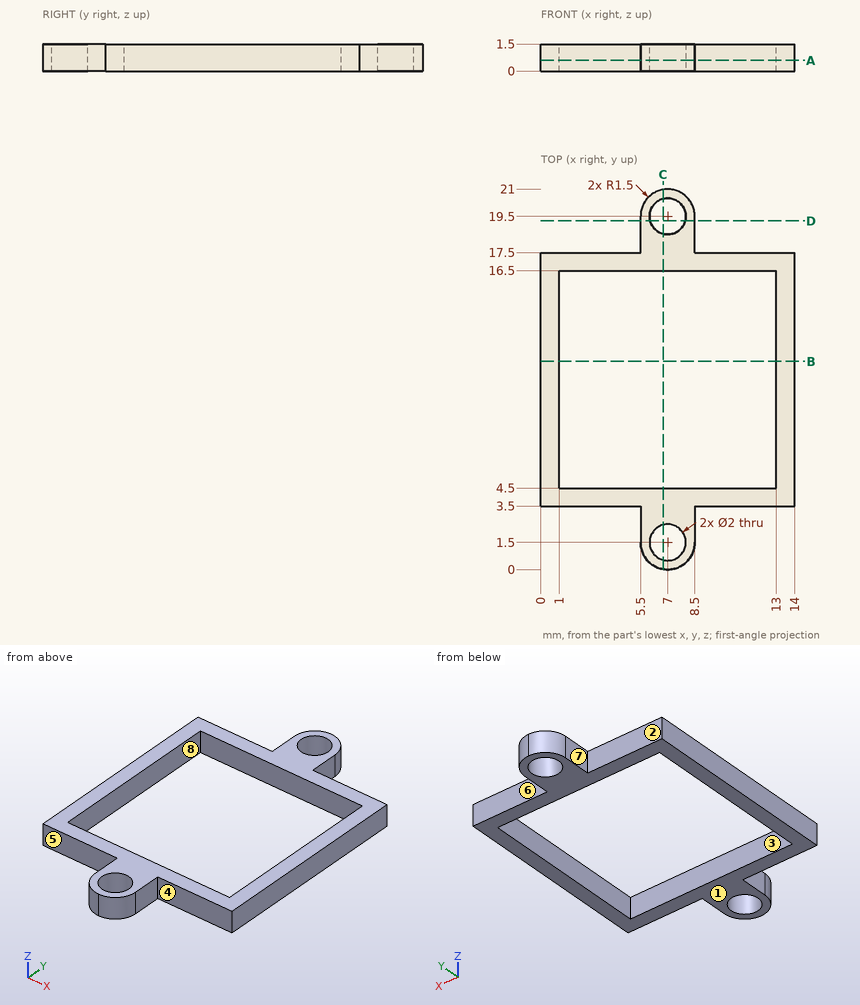
Answer from the drawing. Dimensions are ordinates in mm from the lowest x, y and z of the part. A direction names the side the tool comes from. Round coordinates to 2 decimals unless told otherwise and drop trailing zeros. Loops run counter-clockwise (first coordinate to the right, second up) from the corner with the lowest first, then second, coordinate; pieces in that order, holes last.
(1) Find the intervals of material crossed by L1, parallel to Y at x = 7, z = 0.6; L2, parallel to Y at x = 9.5, z = 0.8; L3, parallel to X at y = 16, z = 0.85, in increasing order.
Computed values:
L1: y = 0 to 0.5, 2.5 to 4.5, 16.5 to 18.5, 20.5 to 21
L2: y = 3.5 to 4.5, 16.5 to 17.5
L3: x = 0 to 1, 13 to 14
(2) The part is cut by section D-D, the plane y = 19.25. Give the vertices of the cut face in (x, z).
Computed values:
outline: (5.5, 0) - (6.03, 0) - (6.03, 1.5) - (5.5, 1.5) - close; (7.97, 0) - (8.5, 0) - (8.5, 1.5) - (7.97, 1.5) - close
(3) The part is cut by section A-A, the plane z = 0.6. Give the vertices of the cut face in (x, y).
Computed values:
outline: (0, 3.5) - (5.5, 3.5) - (5.5, 1.5) arc R1.5 ccw to (8.5, 1.5) - (8.5, 3.5) - (14, 3.5) - (14, 17.5) - (8.5, 17.5) - (8.5, 19.5) arc R1.5 ccw to (5.5, 19.5) - (5.5, 17.5) - (0, 17.5) - close; hole (1, 4.5) - (13, 4.5) - (13, 16.5) - (1, 16.5) - close; hole circle Ø2 at (7, 1.5); hole circle Ø2 at (7, 19.5)
(4) The part is cut by section C-C, the plane x = 6.75. Give the vertices of the cut face in (y, z).
Computed values:
outline: (0.02, 0) - (0.53, 0) - (0.53, 1.5) - (0.02, 1.5) - close; (2.47, 0) - (4.5, 0) - (4.5, 1.5) - (2.47, 1.5) - close; (16.5, 0) - (18.53, 0) - (18.53, 1.5) - (16.5, 1.5) - close; (20.47, 0) - (20.98, 0) - (20.98, 1.5) - (20.47, 1.5) - close
(5) For the marked faces 5, 6, 7 and 8, determine the directions among +Z, -Z, +X, -X, +Y, -Y from which every point of the face is accessible in a straight line to the end or side of a thin tool.
Computed values:
face 5: +Z, -Z, -X, -Y
face 6: +Z, -Z, +X, +Y
face 7: +Z, -Z, -X, +Y
face 8: +Z, -Z
(6) The mould has two halves that part along Y. Classify the marked faces 1, 2, 3 and 4: pulls with the +Y half, pulls with the -Y half, needs draft (parallel to the pull), parting line crosses it, or undercut.
Computed values:
face 1: needs draft
face 2: pulls with the +Y half
face 3: undercut
face 4: pulls with the -Y half
(7) Each of these flat-tipped pins is pushed along its axis until it touches: P1, Ø0.8, axis at x = 4, z = 0.5, coming from the +Y side; P2, Ø0.8, axis at x = 9.5, z = 0.5, coming from the -Y side. Where does it stop, or does it pass through?
Computed values:
P1: stops at y = 17.5
P2: stops at y = 3.5
(8) The part is cut by section B-B, the plane y = 11.5. Give the vertices of the cut face in (x, z).
Computed values:
outline: (0, 0) - (1, 0) - (1, 1.5) - (0, 1.5) - close; (13, 0) - (14, 0) - (14, 1.5) - (13, 1.5) - close
